from build123d import *

# Parameters (mm, degrees)
PAD001_DEPTH         = 9
POCKET001_DEPTH      = 7
SKETCH004_R          = 1.8
POCKET002_DEPTH      = 0.001
POCKET002_DEPTH_BACK = 21.001
SKETCH005_R          = 1.8
POCKET003_DEPTH      = 0.001
POCKET003_DEPTH_BACK = 21.001
POCKET004_DEPTH      = 5
POCKET005_DEPTH      = 5


with BuildPart() as part:
    # Sketch002 → Pad001 (new body, symmetric)
    with BuildSketch(Plane.XZ):
        with BuildLine():
            Line((0, 20), (0, 0))
            Line((0, 0), (20, 0))
            ThreePointArc((20, 0), (20.92388, 0.617317), (20.707107, 1.707107))
            Line((1.707107, 20.707107), (20.707107, 1.707107))
            ThreePointArc((1.707107, 20.707107), (0.617317, 20.92388), (0, 20))
        make_face()
    extrude(amount=PAD001_DEPTH, both=True)

    # Sketch003 → Pocket001 (cut, symmetric)
    with BuildSketch(Plane.XZ):
        Polygon((4, 24), (4, 4), (24, 4), align=None)
    extrude(amount=POCKET001_DEPTH, both=True, mode=Mode.SUBTRACT)

    # Sketch004 → Pocket002 (cut, two sides)
    with BuildSketch(Plane.XY) as pocket002_sk:
        with Locations((12, 0)):
            Circle(SKETCH004_R)
    extrude(amount=-POCKET002_DEPTH, mode=Mode.SUBTRACT)
    extrude(pocket002_sk.sketch, amount=POCKET002_DEPTH_BACK, mode=Mode.SUBTRACT)

    # Sketch005 → Pocket003 (cut, two sides)
    with BuildSketch(Plane.YZ) as pocket003_sk:
        with Locations((0, 12)):
            Circle(SKETCH005_R)
    extrude(amount=-POCKET003_DEPTH, mode=Mode.SUBTRACT)
    extrude(pocket003_sk.sketch, amount=POCKET003_DEPTH_BACK, mode=Mode.SUBTRACT)

    # Sketch006 → Pocket004 (cut)
    with BuildSketch(Plane.YZ.offset(2)):
        Polygon((0, 14.75), (-2.38157, 13.375), (-2.38157, 10.625), (0, 9.25), (2.38157, 10.625), (2.38157, 13.375), align=None)
    extrude(amount=POCKET004_DEPTH, mode=Mode.SUBTRACT)

    # Sketch007 → Pocket005 (cut)
    with BuildSketch(Plane.XY.offset(2)):
        Polygon((14.75, 0), (13.375, 2.38157), (10.625, 2.38157), (9.25, 0), (10.625, -2.38157), (13.375, -2.38157), align=None)
    extrude(amount=POCKET005_DEPTH, mode=Mode.SUBTRACT)


solid = part.part
The model under review builds one solid part; all positions refer to its coordinate system, in mm. A direction names the side the tool comes from. Give positions to 0.01 mm unless a question says otherwise; leave off trailing zeros. Order: outer loops, then holes, each group sorted by start corner. A loop starts at its lowest first (then second) coordinate and runs counter-clockwise, first axis right, second up. Notation, with made-up numbers: M 50.5,77 L 60.5,77 A17 cw 60.5,93 Z; hole C 2.25,11.25 d1. An arc over 180 degrees is marked long. Use one line per item in the form item = value. Start each with the question number.
Item 1: We need section D-D on x = 5.25. Give the boundary of the cut face in (y, z).
Item 2: Insertion check: pin 1 Ø6 at (x, z) = (18, 6.5) entering from +Y; pin 2 Ø2 at (x, y) = (12, 0) entering from +Z; pin 3 Ø6 at (y, z) = (0, 12) entering from +X. Each pin has a flat end and moves straight along its axis. Give the tip position at first contact, or say it passes through.
Item 3: To check wall thickness, follow line 1 along Y through (x, z) = (10.5, 5.25); line 2 along Y through (x, z) = (0.5, 12); line 3 along Z through (x, y) = (12, 2.5). State the ranges of each line that lie inside material, in increasing order. Write a range as from..to.
Item 4: We need section A-A on x = 12. Give the boundary of the cut face in (y, z).
Item 5: We need section C-C on y = -1.5. Give the boundary of the cut face in (x, z).
Item 6: We need section B-B on z = 12. Give the boundary of the cut face in (x, y), plus the area to 3 significant figures.
Item 7: The part is to be moulded in two halves that separate along Z. For faces 1 (the flat face through (11.074, 7.874, 11.34)), 2 (the flat face through (2.99, -1.21, 9.95)), 3 (the flat face through (0, 0, 10)), say which applies: pulls with the +Z half, pulls with the -Z half, needs draft (parallel to the pull), parting line crosses it, or undercut.
Item 8: For faces 4 (the flat face through (3, 2.382, 12)), 5 (the flat face through (14.05, -1.21, 2.99)), 6 (the flat face through (8, -7, 8)), 7 (the cylindrical face through (21, 0, 1)), 8 (the cylindrical face through (1, 0, 21)), list the 3-axis set-ups (+Z, -Z, +X, -X, +Y, -Y) from which the entire face can be reached by the end or side of a thin tool; tool diameter is ignored.
Completed:
q1.outline = M -9,0 L 9,0 L 9,17.16 L 7,17.16 L 7,4 L -7,4 L -7,17.16 L -9,17.16 Z
q2.pin_1 = 9
q2.pin_2 = through
q2.pin_3 = 4
q3.line_1 = -9..-7, 7..9
q3.line_2 = -9..-1.8, 1.8..9
q3.line_3 = 0..4
q4.outline = M -9,0 L -1.8,0 L -1.8,2 L -2.38,2 L -2.38,4 L -7,4 L -7,10.41 L -9,10.41 Z; M 1.8,0 L 9,0 L 9,10.41 L 7,10.41 L 7,4 L 2.38,4 L 2.38,2 L 1.8,2 Z
q5.outline = M 0,0 L 11.01,0 L 11.01,2 L 10.12,2 L 10.12,4 L 4,4 L 4,10.12 L 2,10.12 L 2,11.01 L 0,11.01 Z; M 0,12.99 L 2,12.99 L 2,13.88 L 4,13.88 L 4,18.41 L 1.71,20.71 A1 ccw 0,20 Z; M 12.99,0 L 20,0 A1 ccw 20.71,1.71 L 18.41,4 L 13.88,4 L 13.88,2 L 12.99,2 Z
q6.outline = M 0,-9 L 10.41,-9 L 10.41,-7 L 4,-7 L 4,-2.38 L 2,-2.38 L 2,-1.8 L 0,-1.8 Z; M 0,1.8 L 2,1.8 L 2,2.38 L 4,2.38 L 4,7 L 10.41,7 L 10.41,9 L 0,9 Z
q6.area = 80.9 mm²
q7.face_1 = pulls with the +Z half
q7.face_2 = undercut
q7.face_3 = needs draft
q8.face_4 = +X
q8.face_5 = +Z
q8.face_6 = +Z, +X
q8.face_7 = +X, +Y, -Y
q8.face_8 = +Z, +Y, -Y
